from build123d import *

# Parameters (mm, degrees)
F0_W         = 203.2
F0_H         = 254
F0_R         = 25.4
F1_DEPTH     = 50.8
F2_R         = 6.35
F3_T1_DEPTH  = 53.975
F3_T3_DEPTH  = 60.325
F3_S7_W      = 6.477
F3_S7_H      = 6.477
F3_T8_DEPTH  = 6.477
F3_S13_W     = 6.477
F3_S13_H     = 6.477
F3_T14_DEPTH = 6.477


# Not quite as in the source:
# - a fillet or chamfer that OpenCascade refuses, or shapes differently, is made with other operations: its cross-section is extruded or revolved along the edge and cut away or added


with BuildPart() as f1:
    # F0 (on Top) → F1 (new body)
    with BuildSketch(Plane.XY):
        with Locations((101.6, 127)):
            Rectangle(F0_W, F0_H)
        with Locations((88.8597142273, 50.8)):
            Circle(F0_R, mode=Mode.SUBTRACT)
        with Locations((88.8597142273, 203.2)):
            Circle(F0_R, mode=Mode.SUBTRACT)
    extrude(amount=F1_DEPTH)

    # F2
    f2_edges = [f1.edges().sort_by_distance(p)[0] for p in [
        (0, 127, 0),
        (0, 127, 50.8),
        (101.6, 254, 50.8),
        (63.459714, 203.2, 50.8),
        (63.459714, 50.8, 50.8),
        (101.6, 254, 0),
        (0, 254, 25.4),
        (203.2, 254, 25.4),
        (63.459714, 203.2, 0),
        (63.459714, 50.8, 0),
        (101.6, 0, 0),
        (203.2, 127, 0),
    ]]
    fillet(f2_edges, radius=F2_R)

    # F3: fillet of radius 6.35 on 6 edges, made by hand

    # F3_s2 → F3_t1 (cut)
    with BuildSketch(Plane.XY.offset(6.35)):
        with BuildLine():
            ThreePointArc((0, 6.35), (1.8598719395, 1.8598719395), (6.35, 0))
            Line((6.35, 0), (0, 0))
            Line((0, 0), (0, 6.35))
        make_face()
    extrude(amount=F3_T1_DEPTH, mode=Mode.SUBTRACT)

    # F3_s4 → F3_t3 (cut)
    with BuildSketch(Plane.XY.offset(6.35)):
        with BuildLine():
            ThreePointArc((196.85, 0), (201.3401280605, 1.8598719395), (203.2, 6.35))
            Line((203.2, 6.35), (203.2, 0))
            Line((203.2, 0), (196.85, 0))
        make_face()
    extrude(amount=F3_T3_DEPTH, mode=Mode.SUBTRACT)


with BuildPart() as f3_tool6:
    # F3_s7 → F3_t8 (new body)
    with BuildSketch(Plane.YZ.offset(6.35)):
        with Locations((3.1115, 3.1115)):
            Rectangle(F3_S7_W, F3_S7_H)
    extrude(amount=-F3_T8_DEPTH)

    # F3_s9 → F3_t10 (revolve, cut)
    with BuildSketch(Plane(origin=(6.35, 6.35, 6.35), x_dir=(0, 0.7071067812, 0.7071067812), z_dir=(0, -0.7071067812, 0.7071067812))):
        with BuildLine():
            ThreePointArc((0, -6.35), (6.35, 0), (0, 6.35))
            Line((0, 6.35), (0, -6.35))
        make_face()
    revolve(axis=Axis((6.35, 6.35, 6.35), (-1, 0, 0)), mode=Mode.SUBTRACT)


with BuildPart() as f1_1:
    add(f1.part)

    # F3_t5: cut F3_tool6
    add(f3_tool6.part, mode=Mode.SUBTRACT)


with BuildPart() as f3_tool12:
    # F3_s13 → F3_t14 (new body)
    with BuildSketch(Plane.XZ.offset(-6.35)):
        with Locations((200.0885, 3.1115)):
            Rectangle(F3_S13_W, F3_S13_H)
    extrude(amount=F3_T14_DEPTH)

    # F3_s15 → F3_t16 (revolve, cut)
    with BuildSketch(Plane(origin=(196.85, 6.35, 6.35), x_dir=(-0.7071067812, 0, 0.7071067812), z_dir=(0.7071067812, 0, 0.7071067812))):
        with BuildLine():
            ThreePointArc((0, -6.35), (6.35, 0), (0, 6.35))
            Line((0, 6.35), (0, -6.35))
        make_face()
    revolve(axis=Axis((196.85, 6.35, 6.35), (0, -1, 0)), mode=Mode.SUBTRACT)


with BuildPart() as f1_2:
    add(f1_1.part)

    # F3_t11: cut F3_tool12
    add(f3_tool12.part, mode=Mode.SUBTRACT)


solid = f1_2.part
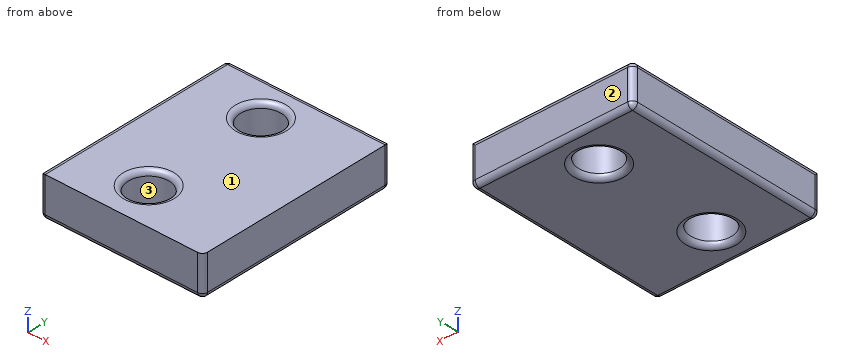
Verification items for the finished model (mm, model axes). Face numbers are marked on the shaded views. Coordinates: 2 decimals unless noted, no trailing zeros. Loops run counter-clockwise (first coordinate to the right, second up) from the corner with the lowest first, then second, coordinate; pieces in that order, holes last. Notation, with made-up numbers: (44.5, 54) -> (99.5, 54) arc R16 cw to (99.5, 66) -> close; hole circle Ø6 at (-15.75, 16). An arc over 180 degrees is marked (long way). Answer as a JSON object with one key per item and string values. Group by question number.
Item 1: Sectioned sample at B-B on y = 50.8. Record the boundary of the cut face in (x, z).
Item 2: Depth check by flat-ended pin: pin 1 (1.5 mm diameter, centred on x = 136.5, z = 20.5, fed in from -Y). Enter the tip coordinate at first touch or a pass-through.
Item 3: Sectioned sample at A-A on z = 11. Record the boundary of the cut face in (x, y).
Item 4: Sectioned sample at C-C on x = 99.5. State how many separate pieces and enclosed holes the cut face has, plus the area to 3 significant figures.
Item 5: Scan lines: probe 1 along Y at (x, z) = (90, 10); probe 2 along Y at (x, z) = (73, 27.5); probe 3 along X at (y, z) = (50, 29). Record each from-to range of solid material in increasing order.
Item 6: Mould release check, pull along Y, two halves, no side actions. Record for the marked faces 1, 2 and 3: +Y half, -Y half, draft (parallel to the pull), parting line (faces both ways), or undercut.
Evaluation:
{
 "1": {"outline": "(0, 6.35) arc R6.35 ccw to (6.35, 0) -> (57.11, 0) arc R6.35 ccw to (63.46, 6.35) -> (63.46, 44.45) arc R6.35 ccw to (57.11, 50.8) -> (6.35, 50.8) arc R6.35 ccw to (0, 44.45) -> close; (114.26, 6.35) arc R6.35 ccw to (120.61, 0) -> (196.85, 0) arc R6.35 ccw to (203.2, 6.35) -> (203.2, 50.8) -> (120.61, 50.8) arc R6.35 ccw to (114.26, 44.45) -> close"},
 "2": {"pin 1": "stops at y = 0"},
 "3": {"outline": "(0, 6.35) arc R6.35 ccw to (6.35, 0) -> (196.85, 0) arc R6.35 ccw to (203.2, 6.35) -> (203.2, 247.65) arc R6.35 ccw to (196.85, 254) -> (6.35, 254) arc R6.35 ccw to (0, 247.65) -> close; hole circle Ø50.8 at (88.86, 50.8); hole circle Ø50.8 at (88.86, 203.2)"},
 "4": {"separate pieces": "3", "enclosed holes": "0", "area": "8,120 mm²"},
 "5": {"probe 1": "y = 0 to 25.43, 76.17 to 177.83, 228.57 to 254", "probe 2": "y = 0 to 30.96, 70.64 to 183.36, 223.04 to 254", "probe 3": "x = 0 to 63.47, 114.25 to 203.2"},
 "6": {"face 1": "draft", "face 2": "+Y half", "face 3": "undercut"}
}
